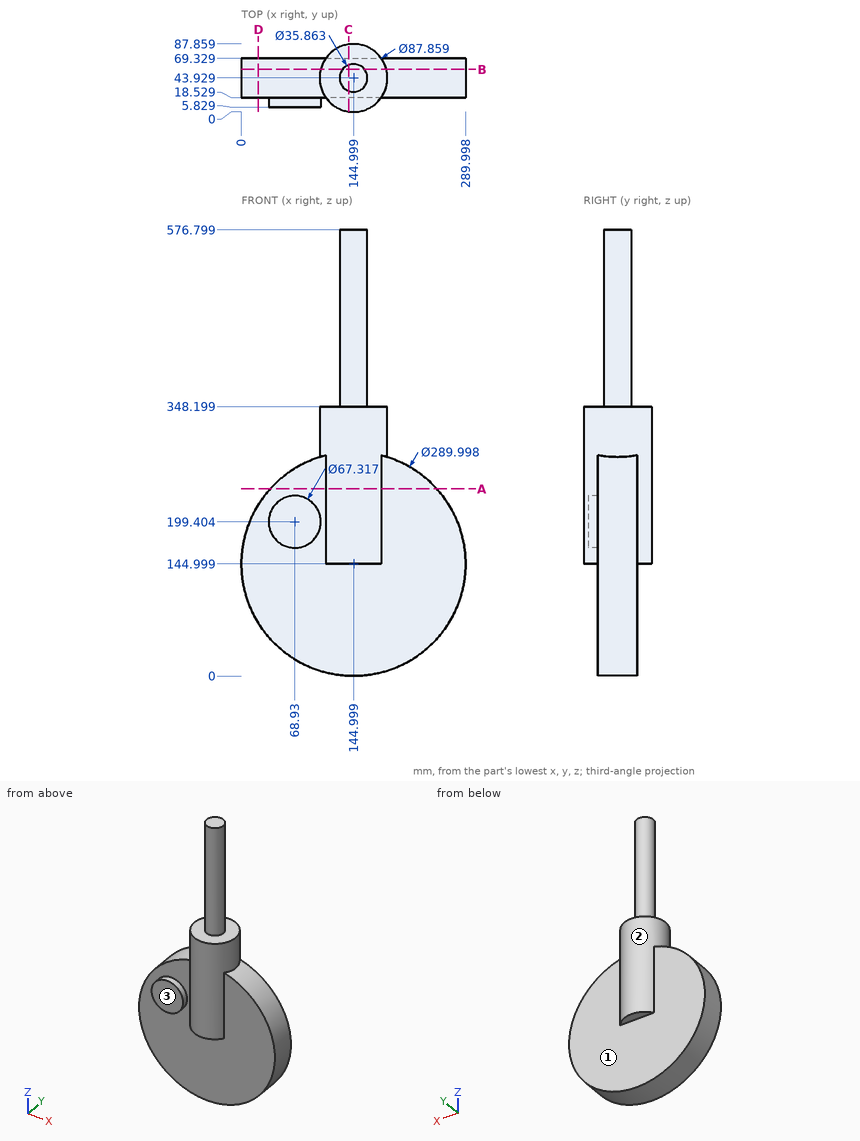
The drawing under review shows one solid part. Ordinate dimensions are in mm from its lowest x, y, z. A direction names the side the tool comes from. Give positions to 0.01 mm unless a question says otherwise; leave off trailing zeros. Write each loop counter-clockwise with the first axis right and the second up, starting at its lowest first coordinate (ties: lowest second). Pieces come first, ordered by that corner, then holes.
1. Add section B-B, the plane y = 55. Write out the cut boundary in (x, z) (1 decimal), plus the area to 3 significant figures.
2. Wall thickness on L1, parallel to Z at x = 144.5, y = 76; L2, parallel to Y at x = 270.5, z = 135.5; L3, parallel to Y at x = 159, z = 313: over which ranges is each line inside the solid? List them lowest first.
3. For P1, Ø15, axis at x = 153, y = 78, coming from the -Z side; P2, Ø5, axis at y = 77, z = 261, coming from the +X side (1 decimal); P3, Ø3, axis at x = 221.5, y = 23.5, coming from the +Z side (1 decimal), all flat-tipped, find the tip position at first contact; note any pin that passes through.
4. Add section C-C, the plane x = 138.5. Write out the cut boundary in (y, z) (1 decimal).
5. Tool access review of the marked faces 1, 2 and 3: name each direction out of +Z, -Z, +X, -X, +Y, -Y from which nothing blocks a thin tool from reaching the whole face with its end or side.
6. Add section A-A, the plane z = 242. Write out the cut boundary in (x, y) (1 decimal).
7. Add section D-D, the plane x = 22. Write out the cut boundary in (y, z) (1 decimal), plus the area to 3 significant figures.
Worked answers:
1. outline: (102.5, 283.6) arc R145 ccw (long way) to (187.5, 283.6) - (187.5, 348.2) - (159.1, 348.2) - (159.1, 576.8) - (130.9, 576.8) - (130.9, 348.2) - (102.5, 348.2) - close
1. area: 77,600 mm2
2. L1: z = 145 to 348.2
2. L2: y = 18.53 to 69.33
2. L3: y = 2.29 to 85.57
3. P1: stops at z = 145
3. P2: stops at x = 176.5
3. P3: stops at z = 269.1
4. outline: (0.5, 145) - (18.5, 145) - (18.5, 0.1) - (69.3, 0.1) - (69.3, 145) - (87.4, 145) - (87.4, 348.2) - (60.6, 348.2) - (60.6, 576.8) - (27.2, 576.8) - (27.2, 348.2) - (0.5, 348.2) - close
5. face 1: -Z, +Y
5. face 2: +Z
5. face 3: +Z, -Z, -X, -Y
6. outline: (37.2, 18.5) - (109.2, 18.5) arc R43.9 ccw to (180.8, 18.5) - (252.8, 18.5) - (252.8, 69.3) - (180.8, 69.3) arc R43.9 ccw to (109.2, 69.3) - (37.2, 69.3) - close
7. outline: (18.5, 68.2) - (69.3, 68.2) - (69.3, 221.8) - (18.5, 221.8) - close
7. area: 7,800 mm2
